from build123d import *

# Parameters (mm, degrees)
CHAMFER1_SIZE      = 1.27
FILLET1_R          = 0.9144
SKETCH3_R          = 1.143
CUT_EXTRUDE1_DEPTH = 2.54
CUT_EXTRUDE2_START = -2.54
SKETCH4_R          = 1.143
CUT_EXTRUDE2_DEPTH = 2.54


with BuildPart() as part:
    # Sketch1 → Revolve1 (revolve)
    with BuildSketch(Plane(origin=(0, 0, 0), x_dir=(0, 0, -1), z_dir=(1, 0, 0)), mode=Mode.PRIVATE) as revolve1_sk:
        Polygon((0, 0), (0, 6.741739825), (2.413, 7.62), (7.493, 7.62), (7.493, 6.0325), (32.893, 6.0325), (32.893, 0), align=None)
    revolve(revolve1_sk.sketch.rotate(Axis((0, 0, -133.35), (0, 0, 1)), 90), axis=Axis((0, 0, -133.35), (0, 0, 1)))

    # Sketch2 → Cut-Revolve1 (revolve, cut)
    with BuildSketch(Plane(origin=(0, 0, 0), x_dir=(0, 0, -1), z_dir=(1, 0, 0)), mode=Mode.PRIVATE) as cut_revolve1_sk:
        with BuildLine():
            Line((7.294796158, 6.342296158), (7.747, 6.7945))
            Line((7.747, 6.7945), (8.255, 6.7945))
            Line((8.255, 6.7945), (8.255, 6.2865))
            Line((8.255, 6.2865), (7.802796158, 5.834296158))
            ThreePointArc((7.802796158, 5.834296158), (7.74099351, 5.793000949), (7.668092316, 5.7785))
            Line((7.668092316, 5.7785), (7.4295, 5.7785))
            ThreePointArc((7.4295, 5.7785), (7.294796158, 5.834296158), (7.239, 5.969))
            Line((7.239, 5.969), (7.239, 6.207592316))
            ThreePointArc((7.239, 6.207592316), (7.253500949, 6.28049351), (7.294796158, 6.342296158))
        make_face()
    revolve(cut_revolve1_sk.sketch.rotate(Axis((0, 0, -133.35), (0, 0, 1)), 90), axis=Axis((0, 0, -133.35), (0, 0, 1)), mode=Mode.SUBTRACT)

    # Chamfer1
    chamfer1_edges = [part.edges().sort_by_distance(p)[0] for p in [
        (6.0325, 0, -32.893),
    ]]
    chamfer(chamfer1_edges, length=CHAMFER1_SIZE)

    # Fillet1
    fillet1_edges = [part.edges().sort_by_distance(p)[0] for p in [
        (6.741739825, 0, 0),
    ]]
    fillet(fillet1_edges, radius=FILLET1_R)

    # Sketch3 → Cut-Extrude1 (cut)
    with BuildSketch(Plane.XY):
        Circle(SKETCH3_R)
    extrude(amount=-CUT_EXTRUDE1_DEPTH, mode=Mode.SUBTRACT)

    # Sketch4 → Cut-Extrude2 (cut)
    with BuildSketch(Plane(origin=(0, 0, -32.893), x_dir=(-1, 0, 0), z_dir=(0, 0, -1)).offset(CUT_EXTRUDE2_START)):
        with Locations(Location((0, 0, 0), (0, 0, 180))):
            Circle(SKETCH4_R)
    extrude(amount=CUT_EXTRUDE2_DEPTH, mode=Mode.SUBTRACT)


solid = part.part
Here's how the part is built. I have some questions about the finished solid (model axes, mm). A direction names the side the tool comes from. Coordinates: 2 decimals unless noted, no trailing zeros. Write each loop counter-clockwise with the first axis right and the second up, starting at its lowest first coordinate (ties: lowest second). Pieces come first, ordered by that corner, then holes.
1) If we section it at A-A (z = -26): List the corners of the cut face in (x, y) for me (1 decimal).
Filled in:
outline: circle Ø12.1 at (0, 0)
2) If I drill on line 1 (Y direction, x = 0, z = -31.3); line 2 (Y direction, x = 0, z = -32.1); line 3 (Y direction, x = 3.75, z = -16), over which ranges is the centre line in solid material (lowest first)?
Filled in:
line 1: y = -6.03 to -1.14, 1.14 to 6.03
line 2: y = -5.56 to -1.14, 1.14 to 5.56
line 3: y = -4.73 to 4.73
3) Which directions (+Z, -Z, +X, -X, +Y, -Y) give clear straight access to the entire face, cutting with the end or side of a thin tool? Please do faces 5 (the face through (1.3, -0.1, 0)), 6 (the face through (0, 0, -2.54)), 7 (the face through (-5.754, -1.812, -19.977)).
Filled in:
face 5: +Z, +X, -X, +Y, -Y
face 6: +Z
face 7: -Z
4) I'm going to push flat-ended pins straight in: pin 1 (2 mm diameter, centred on x = 5, z = -11, fed in from -Y); pin 2 (6 mm diameter, centred on y = -5.5, z = -20, fed in from +X); pin 3 (1 mm diameter, centred on y = 3.5, z = -27, fed in from +X). Where does each tip first touch, or does it pass through?
Filled in:
pin 1: stops at y = -4.52
pin 2: stops at x = 5.49
pin 3: stops at x = 5.23
5) Thinking about a two-plate mould opening in X: for faces 1 (the face through (0.527, 1.014, -31.605)), 2 (the face through (0, 0, -30.353)), 3 (the face through (-1, 1, -32.893)), 4 (the face through (0.992, -7.555, -4.989)), which applies, +X half, -X half, draft (parallel to the pull), parting line (faces both ways), or undercut?
Filled in:
face 1: undercut
face 2: undercut
face 3: draft
face 4: parting line
